The drawing under review shows one solid part. Ordinate dimensions are in mm from its lowest x, y, z. A direction names the side the tool comes from. Round coordinates to 2 decimals unless told otherwise and drop trailing zeros. Loops run counter-clockwise (first coordinate to the right, second up) from the corner with the lowest first, then second, coordinate; pieces in that order, holes last. Notation, with made-up numbers: (89.25, 8) -> (125.25, 8) arc R15 cw to (125.25, 23) -> close; hole circle Ø1 at (-34, 36.25). An arc over 180 degrees is marked (long way). Use a Markdown table: item, result. Add a question column.
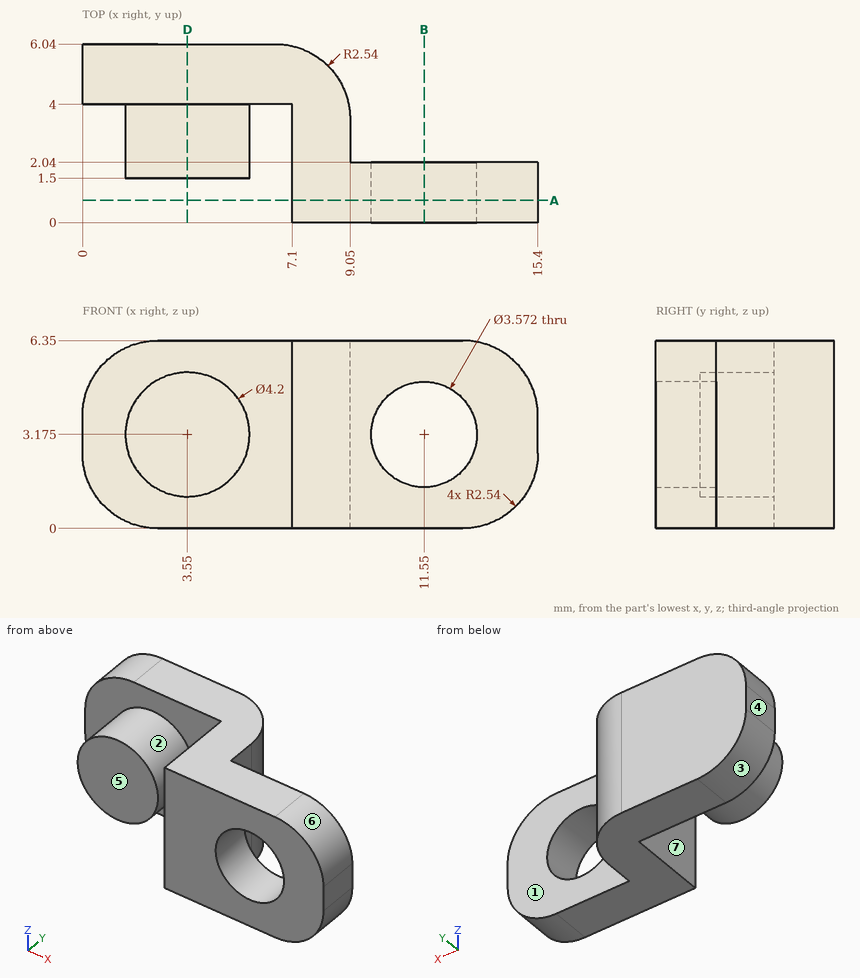
1. Mouldability with a two-part tool opening along X and no side actions: class the marked faces 4, 5, 6 and 7 as +X half, -X half, draft (parallel to the pull), parting line (faces both ways), or undercut.
2. Consider section B-B on x = 11.55. State the section outline as (y, z) points.
3. For the marked faces 1, 2 and 3, list the 3-axis set-ups (+Z, -Z, +X, -X, +Y, -Y) from which the entire face can be reached by the end or side of a thin tool; tool diameter is ignored.
4. To check wall thickness, follow probe 1 along X at (y, z) = (3, 5.5); probe 2 along Y at (x, z) = (4.75, 3); probe 3 along Y at (x, z) = (3, 6). State the ranges of each line that lie inside material, in increasing order. Write a range as from..to.
5. Consider section A-A on y = 0.75. State the section outline as (x, z) points (3 decimals), plus the area to 3 significant figures.
6. Consider section D-D on x = 3.55. State the section outline as (y, z) points (3 decimals).
7. Insertion check: P1, Ø2, axis at y = 2.5, z = 4.5, coming from the -X side; P2, Ø1.9, axis at x = 5, z = 4, coming from the -Y side; P3, Ø0.7, axis at y = 3, z = 3.5, coming from the +X side. Each pin has a flat end and moves straight along its axis. Give the tip position at first contact, or say it passes through.
Verdict:
| question | item | result |
|---|---|---|
| 1 | face 4 | -X half |
| 1 | face 5 | draft |
| 1 | face 6 | +X half |
| 1 | face 7 | undercut |
| 2 | outline | (0, 0) -> (2.04, 0) -> (2.04, 1.39) -> (0, 1.39) -> close; (0, 4.96) -> (2.04, 4.96) -> (2.04, 6.35) -> (0, 6.35) -> close |
| 3 | face 1 | +Z, -Z, +X, +Y |
| 3 | face 2 | -Y |
| 3 | face 3 | -Z, -X, +Y, -Y |
| 4 | probe 1 | x = 7.1..9.05 |
| 4 | probe 2 | y = 1.5..6.04 |
| 4 | probe 3 | y = 4..6.04 |
| 5 | outline | (7.1, 0) -> (12.86, 0) arc R2.54 ccw to (15.4, 2.54) -> (15.4, 3.81) arc R2.54 ccw to (12.86, 6.35) -> (7.1, 6.35) -> close; hole circle Ø3.572 at (11.55, 3.175) |
| 5 | area | 39.9 mm² |
| 6 | outline | (1.5, 1.075) -> (4, 1.075) -> (4, 0) -> (6.04, 0) -> (6.04, 6.35) -> (4, 6.35) -> (4, 5.275) -> (1.5, 5.275) -> close |
| 7 | P1 | stops at x = 1.48 |
| 7 | P2 | stops at y = 1.5 |
| 7 | P3 | stops at x = 9.05 |
